For this review, take the finished solid that the model builds, in its own axes (mm). Face numbers are marked on the shaded views. A direction names the side the tool comes from. Coordinates: 2 decimals unless noted, no trailing zeros. Order: outer loops, then holes, each group sorted by start corner. A loop starts at its lowest first (then second) coordinate and runs counter-clockwise, first axis right, second up.
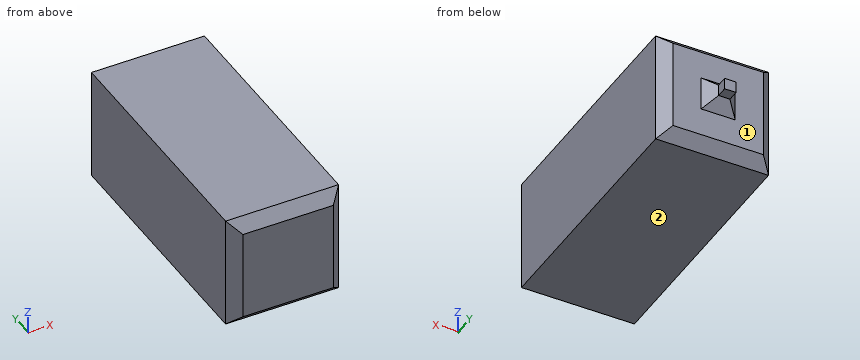
from build123d import *

# Parameters (mm, degrees)
SKETCH1_W           = 500
SKETCH1_H           = 500
BOSS_EXTRUDE1_DEPTH = 1200
SKETCH2_W           = 50.59676849
SKETCH2_H           = 50.59676849
BOSS_EXTRUDE2_DEPTH = 100
CHAMFER1_SIZE       = 50


with BuildPart() as part:
    # Sketch1 → Boss-Extrude1 (new body)
    with BuildSketch(Plane(origin=(0, 0, 0), x_dir=(1, 0, 0), z_dir=(0, 1, 0))):
        Rectangle(SKETCH1_W, SKETCH1_H)
    extrude(amount=BOSS_EXTRUDE1_DEPTH)

    # Sketch2 → Boss-Extrude2 (add)
    with BuildSketch(Plane(origin=(0, 1200, 0), x_dir=(1, 0, 0), z_dir=(0, 1, 0))):
        Rectangle(SKETCH2_W, SKETCH2_H)
    extrude(amount=BOSS_EXTRUDE2_DEPTH)

    # Chamfer1
    chamfer1_edges = [part.edges().sort_by_distance(p)[0] for p in [
        (-250, 1200, 0),
        (25.298384245, 1200, 0),
        (0, 1200, -25.298384245),
        (-25.298384245, 1200, 0),
        (0, 1200, 250),
        (0, 1200, 25.298384245),
        (250, 1200, 0),
        (0, 0, 250),
        (-250, 0, 0),
        (0, 0, -250),
        (250, 0, 0),
        (0, 1200, -250),
    ]]
    chamfer(chamfer1_edges, length=CHAMFER1_SIZE)


solid = part.part
1. Take a section at A-A, the plane x = -216. Give the boundary of the cut face in (y, z).
Answer below:
outline: (16, -216) - (50, -250) - (1150, -250) - (1184, -216) - (1184, 216) - (1150, 250) - (50, 250) - (16, 216) - close
2. Machinability: for the marked faces 1 and 2, which of the approach directions +Z, -Z, +X, -X, +Y, -Y give a long, thin tool a straight path to every point of the face, cutting with its end or side? Answer none if there is none.
Answer below:
face 1: +Y
face 2: -Z, +X, -X, +Y, -Y
3. Take a section at B-B, the plane z = -175. Give the boundary of the cut face in (x, y).
Answer below:
outline: (-250, 50) - (-200, 0) - (200, 0) - (250, 50) - (250, 1150) - (200, 1200) - (-200, 1200) - (-250, 1150) - close
4. Clearance check with flat-ended pins moving along their axes: pin 1 Ø3 at (x, z) = (-4, -65) entering from +Y; pin 2 Ø25 at (x, y) = (-11.5, 1267.5) entering from +Z; pin 3 Ø8 at (x, z) = (-120.5, -44.5) entering from +Y. State where each tip first meets the part, or that it passes through.
Answer below:
pin 1: stops at y = 1211.8
pin 2: stops at z = 25.3
pin 3: stops at y = 1200
5. Take a section at D-D, the plane x = 40. Give the boundary of the cut face in (y, z), plus the area to 3 significant figures.
Answer below:
outline: (0, -200) - (50, -250) - (1150, -250) - (1200, -200) - (1200, -75.3) - (1235.3, -40) - (1235.3, 40) - (1200, 75.3) - (1200, 200) - (1150, 250) - (50, 250) - (0, 200) - close
area: 599,000 mm2
6. To check wall thickness, follow L1, parallel to Y at x = -78.5, z = -138.5; L2, parallel to X at y = 1155, z = 34; L3, parallel to Z at x = -204.5, y = 1169. State the ranges of each line that lie inside material, in increasing order.
Answer below:
L1: y = 0 to 1200
L2: x = -245 to 245
L3: z = -231 to 231
7. Take a section at C-C, the plane z = 62. Give the boundary of the cut face in (x, y), plus the area to 3 significant figures.
Answer below:
outline: (-250, 50) - (-200, 0) - (200, 0) - (250, 50) - (250, 1150) - (200, 1200) - (75.3, 1200) - (62, 1213.3) - (-62, 1213.3) - (-75.3, 1200) - (-200, 1200) - (-250, 1150) - close
area: 597,000 mm2
